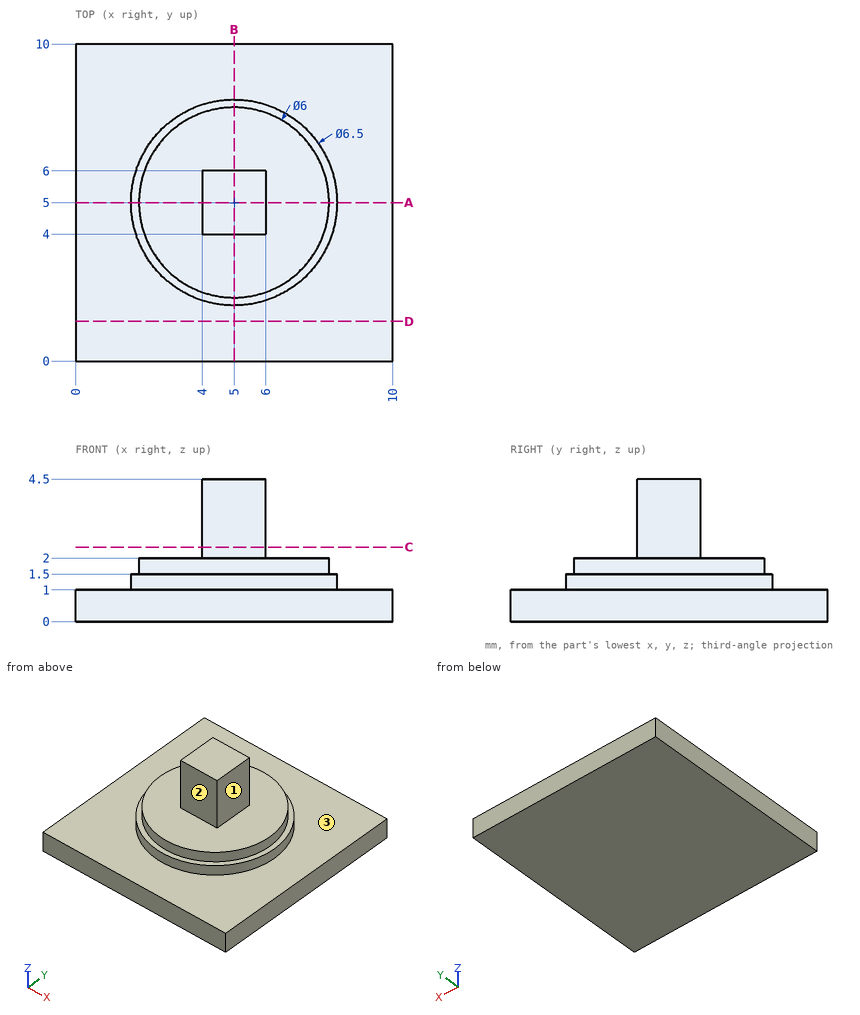
Here's the drawing with two shaded views (mm, measured from the low corner). I have some questions. A direction names the side the tool comes from. Round coordinates to 2 decimals unless told otherwise and drop trailing zeros. Loops run counter-clockwise (first coordinate to the right, second up) from the corner with the lowest first, then second, coordinate; pieces in that order, holes last. Notation, with made-up numbers: (78.25, -21.75) - (96.25, -21.75) arc R24 cw to (96.25, 4.25) - close; hole circle Ø1 at (21.5, -33.5). An arc over 180 degrees is marked (long way). Use CSV: the item, a comma, the result in double quotes.
Item 1: If we section it at C-C on z = 2.35: List the corners of the cut face in (x, y) for me.
Here are the results:
outline,"(4, 4) - (6, 4) - (6, 6) - (4, 6) - close"
Item 2: Will these pins go through, and if not, where does the flat tip stop? pin 1 (1.6 mm diameter, centred on x = 4.5, z = 3.5, fed in from +Y); pin 2 (0.6 mm diameter, centred on x = 5, z = 3, fed in from -Y); pin 3 (1 mm diameter, centred on y = 5, z = 4, fed in from +X).
Here are the results:
pin 1,"stops at y = 6"
pin 2,"stops at y = 4"
pin 3,"stops at x = 6"
Item 3: If we section it at A-A on y = 5: List the corners of the cut face in (x, z) for me, then the cut area to 4 significant figures.
Here are the results:
outline,"(0, 0) - (10, 0) - (10, 1) - (8.25, 1) - (8.25, 1.5) - (8, 1.5) - (8, 2) - (6, 2) - (6, 4.5) - (4, 4.5) - (4, 2) - (2, 2) - (2, 1.5) - (1.75, 1.5) - (1.75, 1) - (0, 1) - close"
area,"21.25 mm²"
Item 4: I need wall thicknesses on L1, parallel to Z at x = 3.5, y = 8.5; L2, parallel to X at y = 4.25, z = 4.25; L3, parallel to Z at x = 7.25, y = 5.5. Which ranges of each line are inside material? Lowest first, please. Write a range as [from, to].
Here are the results:
L1,"z = [0, 1]"
L2,"x = [4, 6]"
L3,"z = [0, 2]"
Item 5: If we section it at D-D on y = 1.25: List the corners of the cut face in (x, z) for me, then the cut area to 3 significant figures.
Here are the results:
outline,"(0, 0) - (10, 0) - (10, 1) - (0, 1) - close"
area,"10.0 mm²"
Item 6: For the marked faces 1, 2 and 3, which set-ups out of +Z, -Z, +X, -X, +Y, -Y let a thin tool reach every point of the face, with its end or its side?
Here are the results:
face 1,"+Z, +X, +Y, -Y"
face 2,"+Z, +X, -X, -Y"
face 3,"+Z"
